Geometry: see drawing. Coordinates: mm, zero at the bounding-box minimum. Round coordinates to 2 decimals unless told otherwise and drop trailing zeros. Write each loop counter-clockwise with the first axis right and the second up, starting at its lowest first coordinate (ties: lowest second). Pieces come first, ordered by that corner, then holes. Notation, with made-up numbers: M -12,4 L 10,4 A17 cw 10,35 Z; hole C 73,6.5 d5. An arc over 180 degrees is marked long. Use one line per item in the form item = value. Start each with the question number.
Item 1: Section query A-A (y = 0.6). Return loops of the section in (x, z), and give its area (3 significant figures).
Item 2: Ray query, probe 1 along Z at (x, y) = (149, 0.5); probe 2 along X at (y, z) = (0.6, 16); probe 3 along Z at (x, y) = (6, 0.45). Return the intervals inside material, ascending.
Item 3: Section query B-B (z = 29). Return loops of the section in (x, y), and give its area (3 significant figures).
Item 4: Section query C-C (x = 118). Return loops of the section in (y, z), and give its area (3 significant figures).
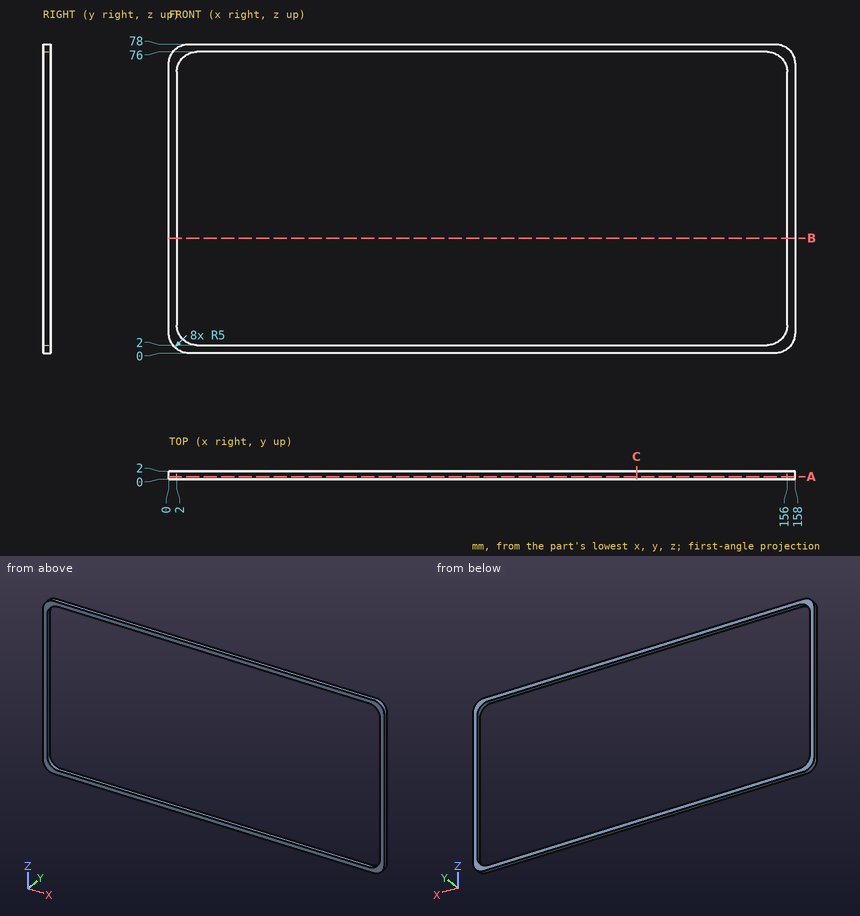
Working result:
q1.outline = M 0,5 A5 ccw 5,0 L 153,0 A5 ccw 158,5 L 158,73 A5 ccw 153,78 L 5,78 A5 ccw 0,73 Z; hole M 2,7 A5 ccw 7,2 L 151,2 A5 ccw 156,7 L 156,71 A5 ccw 151,76 L 7,76 A5 ccw 2,71 Z
q1.area = 928 mm²
q2.probe_1 = 0 to 2, 76 to 78
q2.probe_2 = 0 to 2, 156 to 158
q2.probe_3 = 0 to 2.1, 75.9 to 78
q3.outline = M 0,0 L 2,0 L 2,2 L 0,2 Z; M 156,0 L 158,0 L 158,2 L 156,2 Z
q3.area = 8.00 mm²
q4.outline = M 0,0 L 2,0 L 2,2 L 0,2 Z; M 0,76 L 2,76 L 2,78 L 0,78 Z
q4.area = 8.00 mm²
